Read the model definition and answer for the solid it produces. Units are mm, in the model's axes. Face numbers are marked on the shaded views. Round coordinates to 2 decimals unless told otherwise and drop trailing zeros. Order: outer loops, then holes, each group sorted by start corner. A loop starts at its lowest first (then second) coordinate and runs counter-clockwise, first axis right, second up. Notation, with made-up numbers: (6.25, -38.5) -> (32.25, -38.5) arc R13 cw to (32.25, -32.5) -> close; hole circle Ø1 at (-17, 20). An arc over 180 degrees is marked (long way). Answer as a JSON object with one key per item and string values. Group by question number.
Item 1: Given P1, Ø6, axis at x = -18, y = -46.5, coming from the +Z side; P2, Ø2, axis at x = -75, y = -25, coming from the -Z side; P3, Ø5, axis at x = 33.5, y = -90.5, coming from the -Z side, each flat-ended and moving along its own axis, determine where each tip first touches the part or whether it passes through.
Item 2: Section A-A, the plane x = 0 is taken. Write down the section's boundary in (y, z).
Item 3: Consider probe 1 along X at (y, z) = (-168, 10.5); probe 2 along Z at (x, y) = (3.5, -172.5); probe 3 along X at (y, z) = (-166, 0). Determine where each line is inside the solid, lowest interval first. Write a range as from..to.
Item 4: Section B-B, the plane y = -29 is taken. Count the separate pieces of the cut face and the enclosed holes in it, plus the area to 3 significant figures.
Item 5: The mould has two halves that part along X. Classify the marked faces 1, 2 and 3: pulls with the +X half, pulls with the -X half, needs draft (parallel to the pull), parting line crosses it, or undercut.
Item 6: Section C-C, the plane z = -61.5 is taken. Write down the section's boundary in (x, y).
Item 7: Section D-D, the plane z = -8 is taken. Write down the section's boundary in (x, y), plus the area to 3 significant figures.
from build123d import *

# Parameters (mm, degrees)
F0_R      = 76.2
F1_DEPTH  = 203.2
F2_R      = 12.7
F3_DEPTH  = 38.1
F4_T      = -2.54
F5_W      = 35.56
F5_H      = 7.62
F5_H_2    = 8.0591589212
F6_DEPTH  = 88.9
F7_R      = 12.7
F8_DEPTH  = 241.301
F9_W      = 24.0467190742
F9_H      = 68.9339339733
F9_W_2    = 91.9119119644
F9_H_2    = 9.6131237224
F10_DEPTH = 127


with BuildPart() as f1:
    # F0 (on Front) → F1 (new body)
    with BuildSketch(Plane.XZ):
        Circle(F0_R)
    extrude(amount=F1_DEPTH)

    # F2 (on face) → F3 (join)
    with BuildSketch(Plane.XZ.offset(203.2)):
        Circle(F2_R)
    extrude(amount=F3_DEPTH)

    # F4
    f4_openings = [f1.faces().sort_by_distance(p)[0] for p in [
        (0, 0, 0),
    ]]
    offset(amount=F4_T, openings=f4_openings, kind=Kind.INTERSECTION)

    # F5 (on Right) → F6 (cut, symmetric)
    with BuildSketch(Plane.YZ):
        with Locations((-24.2427656141, 56.4823563671)):
            Rectangle(F5_W, F5_H)
        with Locations((-24.2427656141, 43.4618890285)):
            Rectangle(F5_W, F5_H)
        with Locations((-24.2427656141, 29.6461898834)):
            Rectangle(F5_W, F5_H_2)
        Polygon((-165.2127504349, 65.9124031663), (-191.117182374, 65.9124031663), (-193.4197992086, 54.3993189931), (-193.4197992086, -10.6496037915), (-180.17975986, -10.6496037915), (-180.17975986, 38.2810048759), (-165.2127504349, 52.6723563671), align=None)
    extrude(amount=F6_DEPTH, both=True, mode=Mode.SUBTRACT)

    # F7 (on face) → F8 (cut, through all)
    with BuildSketch(Plane.XZ.offset(241.3)):
        Circle(F7_R)
    extrude(amount=-F8_DEPTH, mode=Mode.SUBTRACT)

    # F9 (on Right) → F10 (cut, symmetric)
    with BuildSketch(Plane.YZ):
        with Locations((-26.3611767441, -32.0650786161)):
            Rectangle(F9_W, F9_H)
        with Locations((-118.2730868459, 4.8065618612)):
            Rectangle(F9_W_2, F9_H_2)
    extrude(amount=F10_DEPTH, both=True, mode=Mode.SUBTRACT)


solid = f1.part
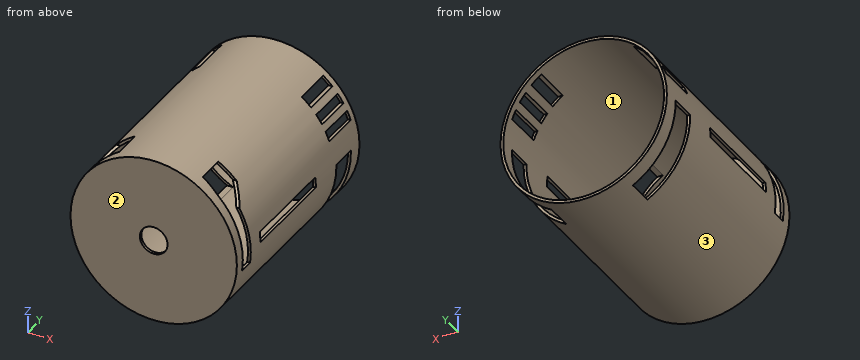
Values found:
{
 "1": {"P1": "z = 74.71", "P2": "z = 2.4", "P3": "z = -69.61"},
 "2": {"outline": "(-203.2, -76.2) -> (0, -76.2) -> (0, -73.66) -> (-200.66, -73.66) -> (-200.66, -12.7) -> (-203.2, -12.7) -> close; (-203.2, 12.7) -> (-200.66, 12.7) -> (-200.66, 73.66) -> (0, 73.66) -> (0, 76.2) -> (-203.2, 76.2) -> close"},
 "3": {"probe 1": "-75.47..-72.91, 72.91..75.47", "probe 2": "-76.12..-73.58, 73.58..76.12", "probe 3": "-76.2..-73.66, 73.66..76.2"},
 "4": {"separate pieces": "8", "enclosed holes": "0", "area": "616 mm2"},
 "5": {"face 1": "undercut", "face 2": "needs draft", "face 3": "parting line crosses it"},
 "6": {"outline": "(-44.99, -203.2) -> (44.99, -203.2) -> (44.99, -38.38) -> (40.54, -38.38) -> (40.54, -200.66) -> (-40.54, -200.66) -> (-40.54, -38.38) -> (-44.99, -38.38) -> close; (-44.99, -14.34) -> (-40.54, -14.34) -> (-40.54, 0) -> (-44.99, 0) -> close; (40.54, -14.34) -> (44.99, -14.34) -> (44.99, 0) -> (40.54, 0) -> close"},
 "7": {"outline": "(-75.78, -203.2) -> (-9.86, -203.2) -> (-9.86, -200.66) -> (-73.22, -200.66) -> (-73.22, -193.42) -> (-75.78, -193.42) -> close; (-75.78, -180.18) -> (-73.22, -180.18) -> (-73.22, -38.38) -> (-75.78, -38.38) -> close; (-75.78, -14.34) -> (-73.22, -14.34) -> (-73.22, 0) -> (-75.78, 0) -> close; (9.86, -203.2) -> (75.78, -203.2) -> (75.78, -193.42) -> (73.22, -193.42) -> (73.22, -200.66) -> (9.86, -200.66) -> close; (73.22, -180.18) -> (75.78, -180.18) -> (75.78, -38.38) -> (73.22, -38.38) -> close; (73.22, -14.34) -> (75.78, -14.34) -> (75.78, 0) -> (73.22, 0) -> close", "area": "1,170 mm2"}
}
